Geometry: final body of the model. Coordinates: model frame, mm. Give positions to 0.01 mm unless a question says otherwise; leave off trailing zeros. Loops run counter-clockwise (first coordinate to the right, second up) from the corner with the lowest first, then second, coordinate; pieces in that order, holes last.
1. Section D-D, the plane x = 38. Output: boundary loops of the cut face in (y, z), then the cut area to 3 significant figures.
2. First-contact query: P1, Ø0.9, axis at x = -8.5, y = 2.5, coming from the -Z side; P2, Ø0.6, axis at x = 13.5, y = 2.5, coming from the -Z side; P3, Ø1.5, axis at y = 2, z = -38, coming from the -X side; P4, Ø1.6, axis at x = -7, z = -28.5, coming from the +Y side. Flat tips, straight axial feed; report the tip coordinate or a pass-through.
3. Section A-A, the plane x = 6. Output: boundary loops of the cut face in (y, z).
4. Section C-C, the plane z = -16.5. Output: boundary loops of the cut face in (x, y).
5. Material intervals for line 1 along X through (y, z) = (2.5, -45); line 2 along X through (y, z) = (1.25, -52); line 3 along X through (y, z) = (0.15, -7.5), sorted ascending.
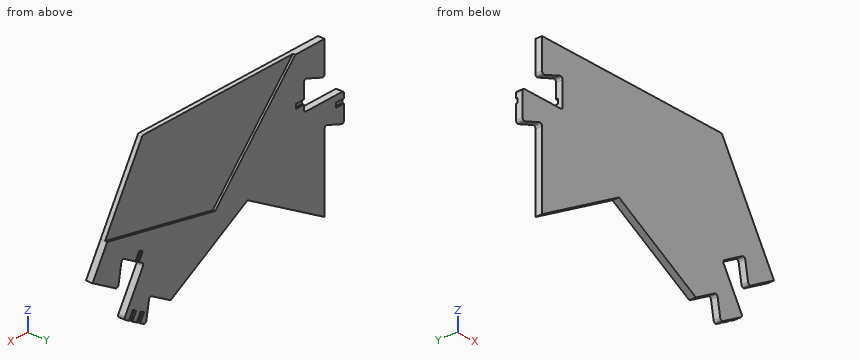
from build123d import *

# Parameters (mm, degrees)
P_IDAT_VYSUNUT_M1_DEPTH  = 3
P_IDAT_VYSUNUT_M2_DEPTH  = 2
ZAOBLIT1_R               = 1
ZAOBLIT2_R               = 1
SKICA2_W                 = 4
SKICA2_H                 = 2
ODEBRAT_VYSUNUT_M1_DEPTH = 0.8


with BuildPart() as part:
    # Skica1 → P_idat vysunut_m1 (new body)
    with BuildSketch(Plane(origin=(0, 0, 0), x_dir=(1, 0, 0), z_dir=(0, 1, 0))):
        Polygon((118.524103266, 46.190077074), (105.53372221, 53.690077074), (103.593400635, 42.685966604), (92.248467845, 49.235966604), (102.473720104, 66.946623035), (91.301992395, 73.396623035), (89.463213481, 62.968389614), (78.635106664, 69.22), (39.317553332, 46.52), (0, 69.22), (0, 33.55662508), (-9.950504516, 37.17831254), (-9.950504516, 24.27831254), (10.5, 24.27831254), (10.5, 11.17831254), (0, 15), (0, 0), (15, 0), (55.910618513, 43.889876884), (111.018549767, 33.190077074), align=None)
    extrude(amount=P_IDAT_VYSUNUT_M1_DEPTH)

    # Skica1_3 → P_idat vysunut_m2 (add)
    with BuildSketch(Plane(origin=(0, 0, 0), x_dir=(1, 0, 0), z_dir=(0, 1, 0))):
        Polygon((91.856249834, 0), (111.018549767, 33.190077074), (55.910618513, 43.889876884), (15, 0), align=None)
    extrude(amount=P_IDAT_VYSUNUT_M2_DEPTH)

    # Zaoblit1
    zaoblit1_edges = [part.edges().sort_by_distance(p)[0] for p in [
        (102.473720104, 1.5, -66.946623035),
        (92.248467845, 1.5, -49.235966604),
        (103.593400635, 1.5, -42.685966604),
        (105.53372221, 1.5, -53.690077074),
        (0, 1.5, -15),
        (10.5, 1.5, -11.17831254),
        (10.5, 1.5, -24.27831254),
        (-9.950504516, 1.5, -24.27831254),
        (-9.950504516, 1.5, -37.17831254),
        (0, 1.5, -33.55662508),
        (89.463213481, 1.5, -62.968389614),
        (91.301992395, 1.5, -73.396623035),
    ]]
    fillet(zaoblit1_edges, radius=ZAOBLIT1_R)

    # Zaoblit2
    zaoblit2_edges = [part.edges().sort_by_distance(p)[0] for p in [
        (91.856249834, 1, 0),
    ]]
    fillet(zaoblit2_edges, radius=ZAOBLIT2_R)

    # Skica2 → Odebrat vysunut_m1 (cut)
    with BuildSketch(Plane(origin=(0, 3, 0), x_dir=(1, 0, 0), z_dir=(0, 1, 0))):
        with Locations((-7.950504516, 28.214238537)):
            Rectangle(SKICA2_W, SKICA2_H)
        with Locations((12.5, 20.242386544)):
            Rectangle(SKICA2_W, SKICA2_H)
        Polygon((94.215365942, 71.714586034), (92.215365942, 68.250484418), (93.947416749, 67.250484418), (95.947416749, 70.714586034), align=None)
        Polygon((96.199082799, 65.950484418), (98.199082799, 69.414586034), (99.931133607, 68.414586034), (97.931133607, 64.950484418), align=None)
        Polygon((96.60970769, 46.718003606), (94.60970769, 43.253901991), (92.877656883, 44.253901991), (94.877656883, 47.718003606), align=None)
    extrude(amount=-ODEBRAT_VYSUNUT_M1_DEPTH, mode=Mode.SUBTRACT)


solid = part.part
Answers below:
1. outline: (0, -47.28) - (3, -47.28) - (3, -24.67) - (2, -24.67) - (2, 0) - (0, 0) - close
1. area: 117 mm2
2. P1: stops at z = -36.75
2. P2: stops at z = -61.6
2. P3: stops at x = 0
2. P4: stops at y = 3
3. outline: (0, -65.76) - (3, -65.76) - (3, -24.28) - (0, -24.28) - close; (0, -12.82) - (3, -12.82) - (3, 0) - (0, 0) - close
4. outline: (10.5, 0) - (101.38, 0) - (101.38, 2) - (30.38, 2) - (30.38, 3) - (10.5, 3) - close
5. line 1: x = 0 to 93.31, 95.62 to 99.59, 104 to 117.84
5. line 2: x = 0 to 29.83, 48.81 to 93.84, 105.24 to 108.46
5. line 3: x = 0 to 96.19
